Geometry: final body of the model. Coordinates: model frame, mm. Round coordinates to 2 decimals unless told otherwise and drop trailing zeros. Write each loop counter-clockwise with the first axis right and the second up, starting at its lowest first coordinate (ties: lowest second). Pieces come first, ordered by that corner, then holes. Notation, with made-up numbers: M 55.5,1.25 L 87.5,1.25 A27 ccw 87.5,27.25 Z; hole C -35.75,-33 d9. An arc over 180 degrees is marked long. Answer as CSV lines item,"result". Start each with the question number.
Q1. Section query B-B on z = -48. Output: boundary loops of the cut face in (x, y), and give its area (3 significant figures).
Q2. Ray query, probe 1 along Z at (x, y) = (-3, 0); probe 2 along X at (y, z) = (-4.5, 6); probe 3 along Y at (x, z) = (3, -48). Return the intervals inside material, ascending.
Q3. First-contact query: pin 1 (6.5 mm diameter, centred on x = 1, z = 46.5, fed in from +Y); pin 2 (3 mm diameter, centred on x = 4, z = 1.5, fed in from -Y); pin 3 (1.8 mm diameter, centred on y = 0, z = -48, fed in from -X); pin 4 (2 mm diameter, centred on x = 3, z = -11, fed in from -Y). Flat tips, straight axial feed; report the tip coordinate or a pass-through.
Q4. Section query A-A on z = -30.5. Output: boundary loops of the cut face in (x, y).
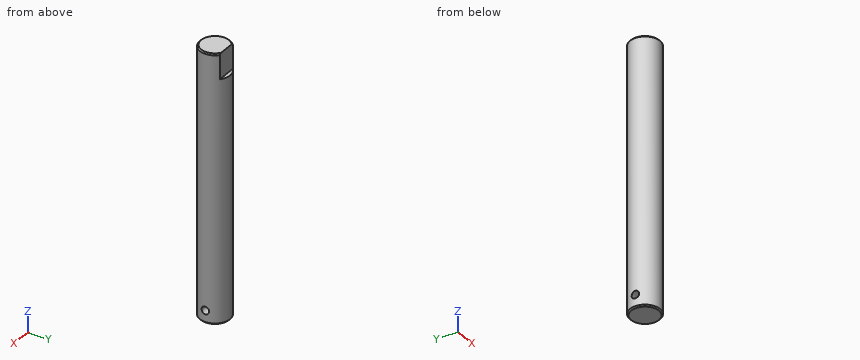
```python
from build123d import *

# Parameters (mm, degrees)
SKETCH1_R              = 6
SHAFT_DEPTH            = 53
HOLE_REACH             = 8
SKETCH2_R              = 1.5
HOLE_DIRECTION_2_REACH = 8
F_0_5X45_CHAMFERS_SIZE = 0.5
FLAT_DEPTH             = 10


with BuildPart() as part:
    # Sketch1 → Shaft (new body, symmetric)
    with BuildSketch(Plane.XY):
        Circle(SKETCH1_R)
    extrude(amount=SHAFT_DEPTH, both=True)

    # Sketch2 → Hole (cut, up to next)
    with BuildSketch(Plane(origin=(0, 0, 0), x_dir=(0, 0, -1), z_dir=(1, 0, 0)), mode=Mode.PRIVATE) as hole_sk1:
        with Locations((48, 0)):
            Circle(SKETCH2_R)
    hole_tool1 = extrude(hole_sk1.sketch, amount=-HOLE_REACH, mode=Mode.PRIVATE) & part.part
    add(hole_tool1.solids().sort_by_distance((0, 0, -48))[0], mode=Mode.SUBTRACT)

    # Sketch2 → Hole direction 2 (cut, up to next)
    with BuildSketch(Plane(origin=(0, 0, 0), x_dir=(0, 0, -1), z_dir=(1, 0, 0)), mode=Mode.PRIVATE) as hole_direction_2_sk1:
        with Locations((48, 0)):
            Circle(SKETCH2_R)
    hole_direction_2_tool1 = extrude(hole_direction_2_sk1.sketch, amount=HOLE_DIRECTION_2_REACH, mode=Mode.PRIVATE) & part.part
    add(hole_direction_2_tool1.solids().sort_by_distance((0, 0, -48))[0], mode=Mode.SUBTRACT)

    # 0.5x45 Chamfers
    f_0_5x45_chamfers_edges = [part.edges().sort_by_distance(p)[0] for p in [
        (-6, 0, -53),
        (-6, 0, 53),
    ]]
    chamfer(f_0_5x45_chamfers_edges, length=F_0_5X45_CHAMFERS_SIZE)

    # Sketch4 → Flat (cut)
    with BuildSketch(Plane.XY.offset(53)):
        with BuildLine():
            Line((-3.968626967, 4.5), (3.968626967, 4.5))
            ThreePointArc((3.968626967, 4.5), (0, 6), (-3.968626967, 4.5))
        make_face()
    extrude(amount=-FLAT_DEPTH, mode=Mode.SUBTRACT)


solid = part.part
```
Entries:
1,outline,"M -5.81,-1.5 A6 ccw 5.81,-1.5 Z; M -5.81,1.5 L 5.81,1.5 A6 ccw Z"
1,area,"77.5 mm^2"
2,probe 1,"z = -53 to -49.5, -46.5 to 53"
2,probe 2,"x = -3.97 to 3.97"
2,probe 3,"y = -5.2 to -1.5, 1.5 to 5.2"
3,pin 1,"stops at y = 4.5"
3,pin 2,"stops at y = -5.45"
3,pin 3,"passes through"
3,pin 4,"stops at y = -5.66"
4,outline,"C 0,0 d12"
